Geometry: final body of the model. Coordinates: model frame, mm. Face numbers are marked on the shaded views. Coordinates: 2 decimals unless noted, no trailing zeros. Loops run counter-clockwise (first coordinate to the right, second up) from the corner with the lowest first, then second, coordinate; pieces in that order, holes last. Notation, with made-up numbers: (13, -20.75) -> (39, -20.75) arc R26 cw to (39, 9.25) -> close; hole circle Ø2 at (9.5, -24). An arc over 180 degrees is marked (long way). One line per item, written item: value. Start each with the question number.
Item 1: Mould query, pull axis Y, two halves, no side actions, for the marked faces 1, 2 and 3. Classes: +Y half, -Y half, draft (parallel to the pull), parting line (faces both ways), or undercut.
Item 2: Section query A-A on x = 0. Return loops of the section in (y, z).
Item 3: Contact query for flat-ended pins moving along their axis: pin 1 Ø2 at (x, y) = (-28, 7) entering from +Z; pin 2 Ø1.5 at (y, z) = (-28, 90) entering from -X; pin 3 Ø4 at (y, z) = (-31.5, 101.5) entering from -X. Output: stop coordinate, or through.
Item 4: Section query C-C on z = 39.5. Return loops of the section in (x, y), then the cut area to 3 significant figures.
Item 5: Ray query, probe 1 along Y at (x, z) = (0, 68); probe 2 along Z at (x, y) = (-9.5, 4.5); probe 3 along Y at (x, z) = (18.5, 92). Return the intervals inside material, ascending. Write a range as from..to.
from build123d import *

# Parameters (mm, degrees)
F0_R     = 44.425612
F1_DEPTH = 127
F2_R     = 38.311037
F3_DEPTH = 93.30304
F4_R     = 5.08
F5_R     = 5.08


with BuildPart() as f1:
    # F0 (on Top) → F1 (new body)
    with BuildSketch(Plane.XY):
        Circle(F0_R)
    extrude(amount=F1_DEPTH)

    # F2 (on face) → F3 (cut)
    with BuildSketch(Plane.XY.offset(127)):
        Circle(F2_R)
    extrude(amount=-F3_DEPTH, mode=Mode.SUBTRACT)

    # F4
    f4_edges = [f1.edges().sort_by_distance(p)[0] for p in [
        (-44.425612, 0, 127),
    ]]
    fillet(f4_edges, radius=F4_R)

    # F5
    f5_edges = [f1.edges().sort_by_distance(p)[0] for p in [
        (-44.425612, 0, 0),
    ]]
    fillet(f5_edges, radius=F5_R)


solid = f1.part
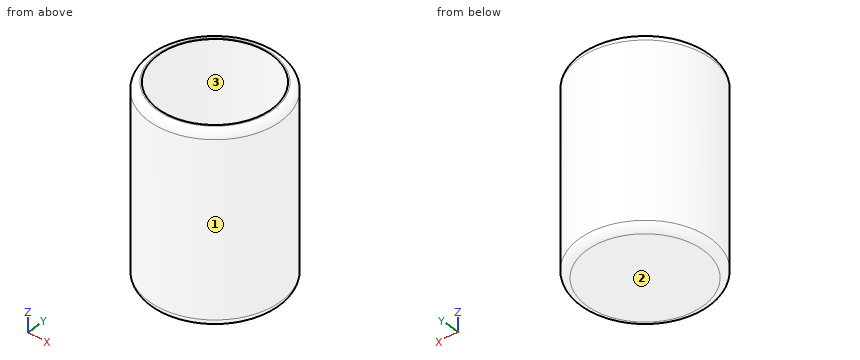
Reply:
1. face 1: parting line
1. face 2: draft
1. face 3: undercut
2. outline: (-44.43, 5.08) arc R5.08 ccw to (-39.35, 0) -> (39.35, 0) arc R5.08 ccw to (44.43, 5.08) -> (44.43, 121.92) arc R5.08 ccw to (39.35, 127) -> (38.31, 127) -> (38.31, 33.7) -> (-38.31, 33.7) -> (-38.31, 127) -> (-39.35, 127) arc R5.08 ccw to (-44.43, 121.92) -> close
3. pin 1: stops at z = 33.7
3. pin 2: stops at x = -35.09
3. pin 3: stops at x = -33.22
4. outline: circle Ø88.85 at (0, 0); hole circle Ø76.62 at (0, 0)
4. area: 1,590 mm²
5. probe 1: y = -44.43..-38.31, 38.31..44.43
5. probe 2: z = 0..33.7
5. probe 3: y = -40.39..-33.55, 33.55..40.39
